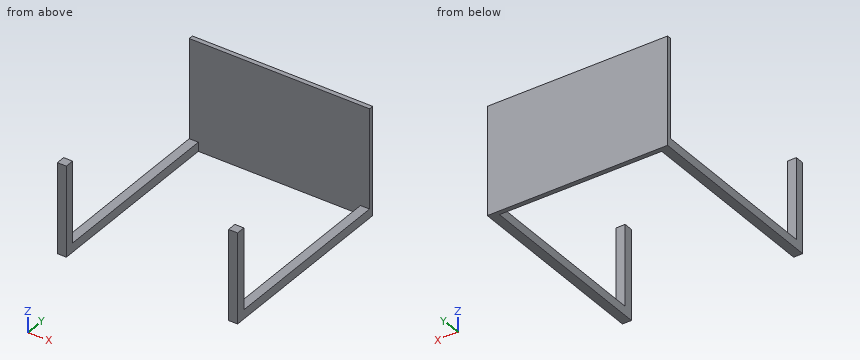
```python
from build123d import *

# Parameters (mm, degrees)
SKETCH1_W           = 1016
SKETCH1_H           = 609.6
BOSS_EXTRUDE1_DEPTH = 25.4
SKETCH2_W           = 50.8
SKETCH2_H           = 50.8
BOSS_EXTRUDE2_DEPTH = 1016
SKETCH3_W           = 50.8
SKETCH3_H           = 508
BOSS_EXTRUDE3_DEPTH = 50.8


with BuildPart() as part:
    # Sketch1 → Boss-Extrude1 (new body)
    with BuildSketch(Plane(origin=(0, 0, 0), x_dir=(1, 0, 0), z_dir=(0, 1, 0))):
        Rectangle(SKETCH1_W, SKETCH1_H)
    extrude(amount=BOSS_EXTRUDE1_DEPTH)

    # Sketch2 → Boss-Extrude2 (add)
    with BuildSketch(Plane(origin=(0, 0, 0), x_dir=(1, 0, 0), z_dir=(0, 1, 0))):
        with Locations((-482.6, 279.4)):
            Rectangle(SKETCH2_W, SKETCH2_H)
        with Locations((482.6, 279.4)):
            Rectangle(SKETCH2_W, SKETCH2_H)
    extrude(amount=-BOSS_EXTRUDE2_DEPTH)

    # Sketch3 → Boss-Extrude3 (add)
    with BuildSketch(Plane(origin=(0, -1016, 0), x_dir=(-1, 0, 0), z_dir=(0, -1, 0))):
        with Locations((482.6, 50.8)):
            Rectangle(SKETCH3_W, SKETCH3_H)
        with Locations((-482.6, 50.8)):
            Rectangle(SKETCH3_W, SKETCH3_H)
    extrude(amount=BOSS_EXTRUDE3_DEPTH)


solid = part.part
```
Geometry: final body of the model. Coordinates: model frame, mm. Round coordinates to 2 decimals unless told otherwise and drop trailing zeros. Write each loop counter-clockwise with the first axis right and the second up, starting at its lowest first coordinate (ties: lowest second). Pieces come first, ordered by that corner, then holes. Notation, with made-up numbers: M 65.25,52.5 L 86.25,52.5 A20 ccw 86.25,72.5 Z; hole C 39,9 d4. An arc over 180 degrees is marked long. Answer in a Markdown table with one row per item. Add a question column.
(1) Cut plane C-C, the plane x = -437.5. Return the cut outline in (y, z), then the cut area to 3 significant figures.
(2) Contact query for flat-ended pins moving along their axis: pin 1 (6 mm diameter, centred on x = -329.5, z = -108, fed in from -Y); pin 2 (15 mm diameter, centred on x = -470, y = -1030.5, fed in from +Z). Output: stop coordinate, or through.
(3) Ray query, L1, parallel to Y at x = 462, z = -127.5; L2, parallel to Y at x = 108, z = -156. Return the intervals inside material, ascending.
(4) Cut plane A-A, the plane z = -195.5. Return the cut outline in (x, y).
(5) Cut plane B-B, the plane y = -64. Return the cut outline in (x, z).
(6) Cut plane D-D, the plane z = 267.5. Return the cut outline in (x, y).
Established:
| question | item | result |
|---|---|---|
| 1 | outline | M 0,-304.8 L 25.4,-304.8 L 25.4,304.8 L 0,304.8 Z |
| 1 | area | 15,500 mm² |
| 2 | pin 1 | y = 0 |
| 2 | pin 2 | z = 203.2 |
| 3 | L1 | -1066.8 to -1016, 0 to 25.4 |
| 3 | L2 | 0 to 25.4 |
| 4 | outline | M -508,-1066.8 L -457.2,-1066.8 L -457.2,-1016 L -508,-1016 Z; M -508,0 L 508,0 L 508,25.4 L -508,25.4 Z; M 457.2,-1066.8 L 508,-1066.8 L 508,-1016 L 457.2,-1016 Z |
| 5 | outline | M -508,-304.8 L -457.2,-304.8 L -457.2,-254 L -508,-254 Z; M 457.2,-304.8 L 508,-304.8 L 508,-254 L 457.2,-254 Z |
| 6 | outline | M -508,0 L 508,0 L 508,25.4 L -508,25.4 Z |
